Can you work these out from the model? Positions are in its coordinate system, mm. A direction names the side the tool comes from. Coordinates: 2 decimals unless noted, no trailing zeros. Order: outer loops, then holes, each group sorted by start corner. A loop starts at its lowest first (then second) coordinate and runs counter-clockwise, first axis right, second up.
```python
from build123d import *

# Parameters (mm, degrees)
F0_W     = 143.039465
F0_H     = 124.044284
F0_R     = 48.455105
F1_DEPTH = 127
F3_DEPTH = 25.4


with BuildPart() as f1:
    # F0 (on Front) → F1 (new body)
    with BuildSketch(Plane.XZ):
        with Locations((-0.719518, 3.021963)):
            Rectangle(F0_W, F0_H)
        Circle(F0_R, mode=Mode.SUBTRACT)
    extrude(amount=F1_DEPTH)

    # F2 (on face) → F3 (cut)
    with BuildSketch(Plane.XY.offset(65.044105)):
        Polygon((35.837892, -101.840705), (0, -34.521569), (-44.855904, -101.840705), align=None)
    extrude(amount=-F3_DEPTH, mode=Mode.SUBTRACT)


solid = f1.part
```
1. Imagine slicing it at B-B on x = 4. Please give me the cut outline in (y, z).
Completed:
outline: (-127, -59) - (0, -59) - (0, -48.29) - (-127, -48.29) - close; (-127, 48.29) - (-101.84, 48.29) - (-101.84, 65.04) - (-127, 65.04) - close; (-42.04, 48.29) - (0, 48.29) - (0, 65.04) - (-42.04, 65.04) - close
2. Please list where these lines run through material, in increasing order: probe 1 along Z at (x, y) = (-39, -106.5); probe 2 along Z at (x, y) = (39.5, -106.5); probe 3 along X at (y, z) = (-97, -8).
Completed:
probe 1: z = -59 to -28.76, 28.76 to 65.04
probe 2: z = -59 to -28.07, 28.07 to 65.04
probe 3: x = -72.24 to -47.79, 47.79 to 70.8
3. Thinking about a two-plate mould opening in Y: for faces 3 (the flat face through (-5, -101.841, 55)), 4 (the flat face through (-2, -63, -59)), 5 (the flat face through (-49, -127, 4)), which applies, pulls with the +Y half, pulls with the -Y half, needs draft (parallel to the pull), parting line crosses it, or undercut?
Completed:
face 3: undercut
face 4: needs draft
face 5: pulls with the -Y half
4. Imagine slicing it at C-C on y = -117.5. Please give me the cut outline in (x, z).
Completed:
outline: (-72.24, -59) - (70.8, -59) - (70.8, 65.04) - (-72.24, 65.04) - close; hole circle Ø96.91 at (0, 0)
5. Imagine slicing it at D-D on x = 38. Please give me the cut outline in (y, z).
Completed:
outline: (-127, -59) - (0, -59) - (0, -30.06) - (-127, -30.06) - close; (-127, 30.06) - (0, 30.06) - (0, 65.04) - (-127, 65.04) - close
6. Imagine slicing it at A-A on z = 0. Please give me the cut outline in (x, y), then the cut area to 3 significant figures.
Completed:
outline: (-72.24, -127) - (-48.46, -127) - (-48.46, 0) - (-72.24, 0) - close; (48.46, -127) - (70.8, -127) - (70.8, 0) - (48.46, 0) - close
area: 5,860 mm2
7. On a 3-axis mill with a long thin cutter (end or side, diameter ignored), from which of +Z, -Z, +X, -X, +Y, -Y can I reach the whole of each face in a straight line? I mean faces 1 (the flat face through (14, -48, 65.044)), 2 (the flat face through (-33, -95, 39.644)). Say none if no direction works.
Completed:
face 1: +Z, +X, -X, +Y, -Y
face 2: +Z
